Answer from the drawing. Dimensions are ordinates in mm from the lowest x, y and z of the part. Round coordinates to 2 decimals unless told otherwise and drop trailing zeros. Write each loop counter-clockwise with the first axis right and the second up, starting at its lowest first coordinate (ties: lowest second). Pieces come first, ordered by that corner, then holes. Notation, with made-up numbers: (-25.75, 88) - (-9.75, 88) arc R16 cw to (-9.75, 93) - close; hole circle Ø5 at (52.25, 5.25). An arc over 180 degrees is marked (long way). Answer as CSV lines item,"result". Start each with the question number.
1) This flat-tipped pin is pushed along its axis until it touches: pin 1 (3.5 mm diameter, centred on y = 5, z = 25, fed in from -X). Where does it stop, or does it pass through?
2) Find section A-A on y = 3. Determine the outline of the cut face in (x, z), then the cut area to 3 significant figures.
3) Consider line 1 along Y through (x, z) = (5.25, 25); line 2 along Z through (x, y) = (4.5, 5); line 3 along Z through (x, y) = (8.25, 3.75). Determine where each line is inside the solid, lowest interval first.
4) Find section C-C on y = 6.75. Determine the outline of the cut face in (x, z), then the cut area to 3 significant figures.
5) For a pull along Y with two mould halves and no side action, classify the marked faces 1, 2 and 3 as +Y half, -Y half, draft (parallel to the pull), parting line (faces both ways), or undercut.
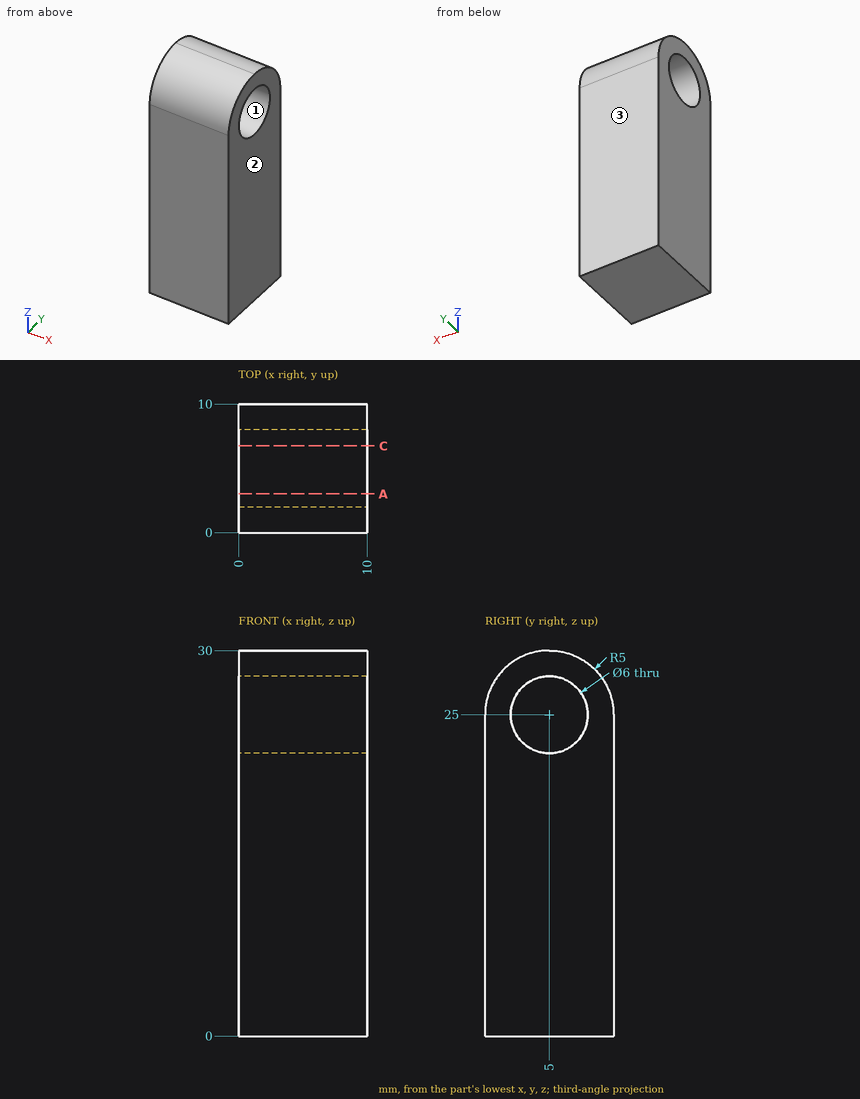
Check values:
1,pin 1,"passes through"
2,outline,"(0, 0) - (10, 0) - (10, 22.76) - (0, 22.76) - close; (0, 27.24) - (10, 27.24) - (10, 29.58) - (0, 29.58) - close"
2,area,"251 mm^2"
3,line 1,"y = 0 to 2, 8 to 10"
3,line 2,"z = 0 to 22, 28 to 30"
3,line 3,"z = 0 to 22.27, 27.73 to 29.84"
4,outline,"(0, 0) - (10, 0) - (10, 22.56) - (0, 22.56) - close; (0, 27.44) - (10, 27.44) - (10, 29.68) - (0, 29.68) - close"
4,area,"248 mm^2"
5,face 1,"undercut"
5,face 2,"draft"
5,face 3,"+Y half"
